from build123d import *

# Parameters (mm, degrees)
F0_W      = 76.2
F0_H      = 177.8
F1_DEPTH  = 19.05
F2_R      = 25.4
F4_DEPTH  = 25.4
F6_DEPTH  = 25.4
F7_W      = 76.2
F7_H      = 15.875
F8_DEPTH  = 12.7
F9_W      = 36.5125
F9_H      = 19.05
F10_DEPTH = 9.525
F11_W     = 12.7
F11_H     = 25.4
F12_DEPTH = 25.4
F13_R     = 34.925
F14_DEPTH = 25.4
F15_W     = 19.05
F15_H     = 38.1
F16_DEPTH = 25.4


with BuildPart() as f1:
    # F0 (on Top) → F1 (new body)
    with BuildSketch(Plane.XY):
        with Locations((-43.904473, 16.184047)):
            Rectangle(F0_W, F0_H)
    extrude(amount=F1_DEPTH)

    # F2
    f2_edges = [f1.edges().sort_by_distance(p)[0] for p in [
        (-5.804473, 105.084047, 9.525),
    ]]
    fillet(f2_edges, radius=F2_R)

    # F3 (on face) → F4 (cut)
    with BuildSketch(Plane.XY.offset(19.05)):
        Polygon((-61.366973, 105.084047), (-82.004473, 105.084047), (-82.004473, 84.446547), align=None)
    extrude(amount=-F4_DEPTH, mode=Mode.SUBTRACT)

    # F5 (on face) → F6 (cut)
    with BuildSketch(Plane.XY.offset(19.05)):
        with BuildLine():
            Line((-31.204473, 105.084047), (-55.016973, 105.084047))
            Line((-55.016973, 105.084047), (-55.016973, 92.384047))
            Line((-55.016973, 92.384047), (-29.616973, 92.384047))
            Line((-29.616973, 92.384047), (-29.616973, 105.034389))
            ThreePointArc((-29.616973, 105.034389), (-30.410334, 105.071629), (-31.204473, 105.084047))
        make_face()
    extrude(amount=-F6_DEPTH, mode=Mode.SUBTRACT)

    # F7 (on face) → F8 (cut)
    with BuildSketch(Plane.XY.offset(19.05)):
        with Locations((-43.904473, -64.778453)):
            Rectangle(F7_W, F7_H)
    extrude(amount=-F8_DEPTH, mode=Mode.SUBTRACT)

    # F9 (on face) → F10 (cut)
    with BuildSketch(Plane.XY.offset(19.05)):
        with Locations((-24.060723, -31.440953)):
            Rectangle(F9_W, F9_H)
    extrude(amount=-F10_DEPTH, mode=Mode.SUBTRACT)

    # F11 (on face) → F12 (cut)
    with BuildSketch(Plane.XY.offset(19.05)):
        with Locations((-12.154473, 16.184047)):
            Rectangle(F11_W, F11_H)
    extrude(amount=-F12_DEPTH, mode=Mode.SUBTRACT)

    # F13 (on face) → F14 (cut)
    with BuildSketch(Plane.XY.offset(19.05)):
        with Locations((-97.879473, -9.215953)):
            Circle(F13_R)
    extrude(amount=-F14_DEPTH, mode=Mode.SUBTRACT)

    # F15 (on face) → F16 (cut)
    with BuildSketch(Plane.XY.offset(19.05)):
        with Locations((-51.841973, 35.234047)):
            Rectangle(F15_W, F15_H)
    extrude(amount=-F16_DEPTH, mode=Mode.SUBTRACT)


solid = f1.part
Work out the finished part from the listing and answer in its coordinate system (mm). A direction names the side the tool comes from. Give positions to 0.01 mm unless a question says otherwise; leave off trailing zeros. Order: outer loops, then holes, each group sorted by start corner. A loop starts at its lowest first (then second) coordinate and runs counter-clockwise, first axis right, second up. Notation, with made-up numbers: M 13,-16.75 L 48,-16.75 A8 ccw 48,-11.75 Z; hole C 43.25,-24 d2. An arc over 180 degrees is marked long. Return JSON: item names as keys, results as strings.
Q1. The mould has two halves that part along Y. Classify faces 5 (the face through (-12.51, 96.88, 9.66)), 6 (the face through (-5.804, -27, 7)), 7 (the face through (-42.317, 35, 10)): pulls with the +Y half, pulls with the -Y half, needs draft (parallel to the pull), parting line crosses it, or undercut.
Answer below:
{"face 5": "pulls with the +Y half", "face 6": "needs draft", "face 7": "undercut"}
Q2. Find section C-C, the plane y = 30.5. Write down the section's boundary in (x, z), and give its area (3 significant figures).
Answer below:
{"outline": "M -82,0 L -61.37,0 L -61.37,19.05 L -82,19.05 Z; M -42.32,0 L -5.8,0 L -5.8,19.05 L -42.32,19.05 Z", "area": "1,090 mm^2"}
Q3. Each of these flat-tipped pins is pushed along its axis until it touches: pin 1 (3 mm diameter, centred on x = -19.5, z = 13, fed in from +Y); pin 2 (9.5 mm diameter, centred on x = -29.5, y = -31, fed in from +Z) (3 decimals); pin 3 (10 mm diameter, centred on x = -37.5, z = 6, fed in from +Y). Where does it stop, or does it pass through?
Answer below:
{"pin 1": "stops at y = 102.94", "pin 2": "stops at z = 9.525", "pin 3": "stops at y = 92.38"}
Q4. Find section B-B, the plane z = 4.25. Write down the section's boundary in (x, y) (3 decimals), and give its area (3 significant figures).
Answer below:
{"outline": "M -82.004,-72.716 L -5.804,-72.716 L -5.804,3.484 L -18.504,3.484 L -18.504,28.884 L -5.804,28.884 L -5.804,79.684 A25.4 ccw -29.617,105.034 L -29.617,92.384 L -55.017,92.384 L -55.017,105.084 L -61.367,105.084 L -82.004,84.447 L -82.004,21.893 A34.925 cw -82.004,-40.324 Z; hole M -61.367,16.184 L -42.317,16.184 L -42.317,54.284 L -61.367,54.284 Z", "area": "11,000 mm^2"}
Q5. Find section D-D, the plane x = -31.5. Write down the section's boundary in (y, z) (3 decimals), and give its area (3 significant figures).
Answer below:
{"outline": "M -72.716,0 L 92.384,0 L 92.384,19.05 L -21.916,19.05 L -21.916,9.525 L -40.966,9.525 L -40.966,19.05 L -56.841,19.05 L -56.841,6.35 L -72.716,6.35 Z", "area": "2,760 mm^2"}
Q6. Find the intervals of material crossed by line 1 along Y through (x, z) = (-42.5, 17.75); line 2 along Y through (x, z) = (-51, 1.75); line 3 along X through (y, z) = (22.5, 17), in increasing order. Write a range as [from, to].
Answer below:
{"line 1": "y = [-56.84, 16.18], [54.28, 92.38]", "line 2": "y = [-72.72, 16.18], [54.28, 92.38]", "line 3": "x = [-82, -61.37], [-42.32, -18.5]"}
Q7. Find section A-A, the plane x = -48. Write down the section's boundary in (y, z).
Answer below:
{"outline": "M -72.72,0 L 16.18,0 L 16.18,19.05 L -56.84,19.05 L -56.84,6.35 L -72.72,6.35 Z; M 54.28,0 L 92.38,0 L 92.38,19.05 L 54.28,19.05 Z"}
Q8. Which of the six approach directions +Z, -Z, +X, -X, +Y, -Y give full straight-line access (tool end or side, diameter ignored) to faces 1 (the face through (-24, -40.966, 14)), 2 (the face through (-12, 28.884, 10)), 3 (the face through (-44, -65, 6.35)), 4 (the face through (-61.367, 35, 10))?
Answer below:
{"face 1": "+Z, +X", "face 2": "+Z, -Z, +X", "face 3": "+Z, +X, -X, -Y", "face 4": "+Z, -Z"}
